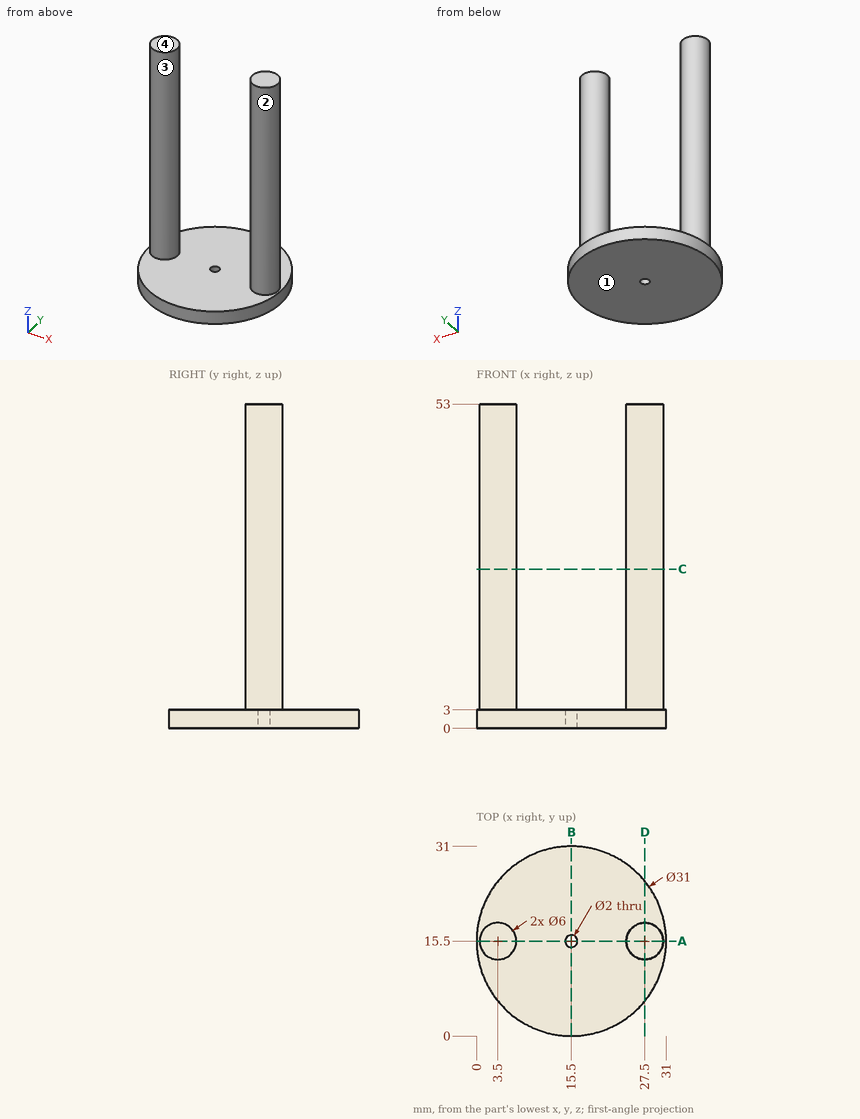
Can you work these out from the drawing? Everything is in mm from the part's minimum corner. A direction names the side the tool comes from. Round coordinates to 2 decimals unless told otherwise and drop trailing zeros. Write each loop counter-clockwise with the first axis right and the second up, starting at its lowest first coordinate (ties: lowest second). Pieces come first, ordered by that corner, then holes. Notation, with made-up numbers: (51, 70) - (101, 70) arc R24 cw to (101, 82) - close; hole circle Ø2 at (-1.5, 11.5). An arc over 180 degrees is marked (long way). Put each result on its own line as item: value. Start each with the question number.
(1) Thinking about a two-plate mould opening in X: for the marked faces 3 and 4, which applies, released by +X, released by -X, zero draft, split by the parting line, or undercut?
(2) I want a section at D-D, the plane x = 27.5. Please give me the cut outline in (y, z).
(3) For the marked faces 1 and 2, which set-ups out of +Z, -Z, +X, -X, +Y, -Y let a thin tool reach every point of the face, with its end or its side?
(4) I need wall thicknesses on probe 1 along Y at (x, z) = (15.5, 0.65); probe 2 along Z at (x, y) = (8, 3.5); probe 3 along X at (y, z) = (18, 9). Which ranges of each line are inside material? Lowest first, please.
(5) Will these pins go through, and if not, where does the flat tip stop? pin 1 (10 mm diameter, centred on x = 25.5, z = 16, fed in from +Y); pin 2 (5 mm diameter, centred on x = 18, y = 24.5, fed in from +Z); pin 3 (5 mm diameter, centred on y = 20, z = 17, fed in from -X).
(6) I want a section at A-A, the plane y = 15.5. Please give me the cut outline in (x, z), plus the area to 3 significant figures.
(7) I want a section at C-C, the plane z = 26. Please give me the cut outline in (x, y).
(8) I want a section at B-B, the plane x = 15.5. Please give me the cut outline in (y, z).
Here are the results:
1. face 3: undercut
1. face 4: zero draft
2. outline: (5.69, 0) - (25.31, 0) - (25.31, 3) - (18.5, 3) - (18.5, 53) - (12.5, 53) - (12.5, 3) - (5.69, 3) - close
3. face 1: -Z, +X, -X, +Y, -Y
3. face 2: +Z
4. probe 1: y = 0 to 14.5, 16.5 to 31
4. probe 2: z = 0 to 3
4. probe 3: x = 1.84 to 5.16, 25.84 to 29.16
5. pin 1: stops at y = 18.5
5. pin 2: stops at z = 3
5. pin 3: stops at x = 1.26
6. outline: (0, 0) - (14.5, 0) - (14.5, 3) - (6.5, 3) - (6.5, 53) - (0.5, 53) - (0.5, 3) - (0, 3) - close; (16.5, 0) - (31, 0) - (31, 3) - (30.5, 3) - (30.5, 53) - (24.5, 53) - (24.5, 3) - (16.5, 3) - close
6. area: 687 mm^2
7. outline: circle Ø6 at (3.5, 15.5); circle Ø6 at (27.5, 15.5)
8. outline: (0, 0) - (14.5, 0) - (14.5, 3) - (0, 3) - close; (16.5, 0) - (31, 0) - (31, 3) - (16.5, 3) - close
